Source: three-view drawing plus pictorial views. Frame: mm from the lowest corner of the part. Give positions to 0.01 mm unless a question says otherwise; leave off trailing zeros. Order: outer loops, then holes, each group sorted by start corner. A loop starts at its lowest first (then second) coordinate and runs counter-clockwise, first axis right, second up. Notation, with made-up numbers: (-0.5, 8.25) -> (47.5, 8.25) arc R27 cw to (47.5, 25.25) -> close; hole circle Ø1 at (64.5, 83). An arc over 180 degrees is marked (long way). Answer in a Markdown table with one row per item. Add a question column.
Q1. Contact query for flat-ended pins moving along their axis: P1, Ø6, axis at x = 7, y = 10.5, coming from the -Z side; P2, Ø4, axis at x = 8.5, z = 57.5, coming from the +Y side; P3, Ø10, axis at x = 7.5, z = 28.5, coming from the -Y side; P4, Ø2, axis at y = 22.5, z = 30, coming from the +X side. Output: stop coordinate, or through.
Q2. Line query: line 1 along Z through (x, y) = (5.25, 5); line 2 along Y through (x, z) = (2.5, 29); line 3 along X through (y, z) = (1.75, 51.5). Output: solid intervals per line, ascending. Write a range as from..to.
Q3. Cut plane B-B on z = 25.5. Return the cut outline in (x, y).
Q4. Cut plane A-A on y = 11.75. Return the cut outline in (x, z), and give its area (3 significant figures).
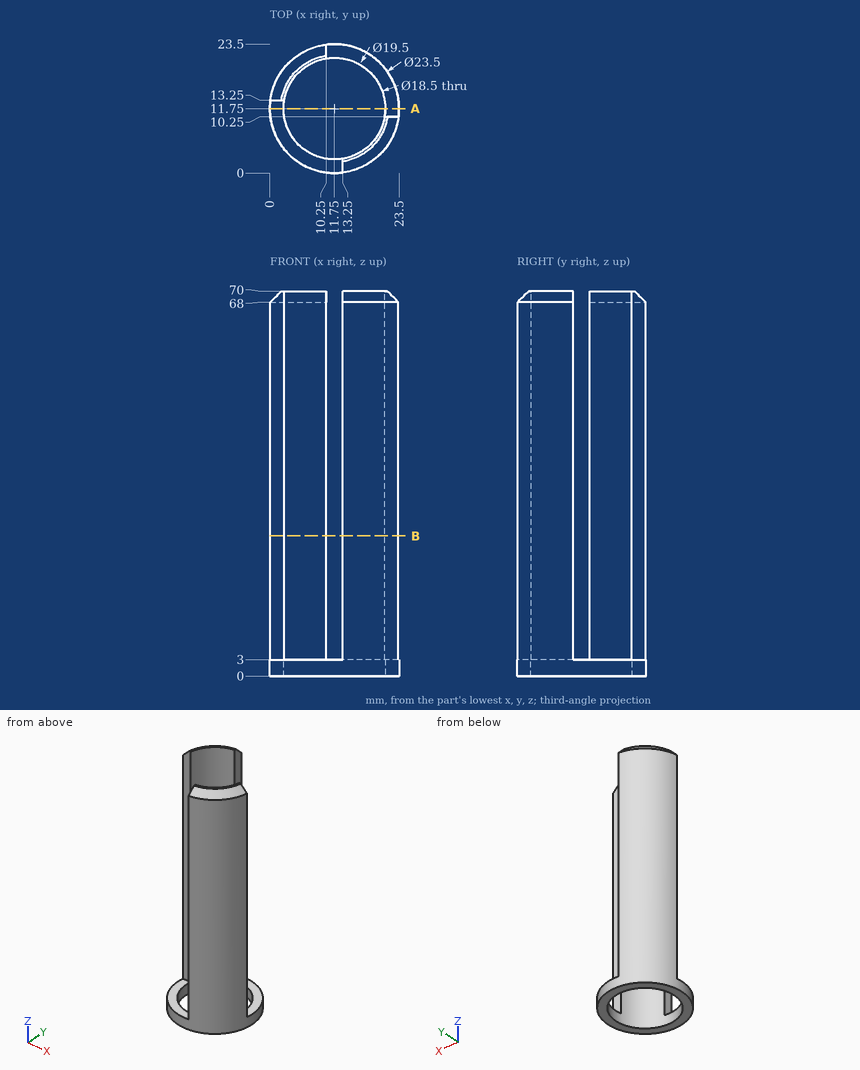
Completed:
| question | item | result |
|---|---|---|
| 1 | P1 | passes through |
| 1 | P2 | stops at y = 23.4 |
| 1 | P3 | stops at y = 13.25 |
| 1 | P4 | stops at x = 10.25 |
| 2 | line 1 | z = 0..3 |
| 2 | line 2 | y = 13.25..19 |
| 2 | line 3 | x = 13.25..17.92 |
| 3 | outline | (0.1, 13.25) -> (2.62, 13.25) arc R9.25 cw to (10.25, 20.88) -> (10.25, 23.4) arc R11.75 ccw to start; (13.25, 0.1) arc R11.75 ccw to (23.4, 10.25) -> (20.88, 10.25) arc R9.25 cw to (13.25, 2.62) -> close |
| 4 | outline | (0, 0) -> (2.5, 0) -> (2.5, 3) -> (0, 3) -> close; (21, 0) -> (23.5, 0) -> (23.5, 3) -> (21, 3) -> close |
| 4 | area | 15.0 mm² |
